Read the model definition and answer for the solid it produces. Units are mm, in the model's axes. Coordinates: 2 decimals unless noted, no trailing zeros. Order: outer loops, then holes, each group sorted by start corner. A loop starts at its lowest first (then second) coordinate and runs counter-clockwise, first axis right, second up. Notation, with made-up numbers: (-16, 62.5) -> (23, 62.5) arc R21 cw to (23, 71.5) -> close; hole circle Ø11 at (54, 34). An arc over 180 degrees is marked (long way). Return JSON: item names as keys, results as strings. Group by question number.
```python
from build123d import *

# Parameters (mm, degrees)
MODEL_R                 = 1.5
SALIENTE_EXTRUIR1_DEPTH = 3


with BuildPart() as part:
    # Model → Saliente-Extruir1 (new body)
    with BuildSketch(Plane.XY):
        with BuildLine():
            Line((-105.943383637, 101.056539338), (-105.943383637, 74.056539338))
            ThreePointArc((-105.943383637, 74.056539338), (-104.625364152, 70.874558823), (-101.443383637, 69.556539338))
            Line((-101.443383637, 69.556539338), (-20.443383637, 69.556539338))
            ThreePointArc((-20.443383637, 69.556539338), (-17.261403122, 70.874558823), (-15.943383637, 74.056539338))
            Line((-15.943383637, 74.056539338), (-15.943383637, 101.056539338))
            ThreePointArc((-15.943383637, 101.056539338), (-17.261403122, 104.238519853), (-20.443383637, 105.556539338))
            Line((-20.443383637, 105.556539338), (-101.443383637, 105.556539338))
            ThreePointArc((-101.443383637, 105.556539338), (-104.625364152, 104.238519853), (-105.943383637, 101.056539338))
        make_face()
        with Locations((-101.443383637, 101.056539338)):
            Circle(MODEL_R, mode=Mode.SUBTRACT)
        with Locations((-92.443383637, 101.056539338)):
            Circle(MODEL_R, mode=Mode.SUBTRACT)
        with Locations((-83.443383637, 101.056539338)):
            Circle(MODEL_R, mode=Mode.SUBTRACT)
        with Locations((-74.443383637, 101.056539338)):
            Circle(MODEL_R, mode=Mode.SUBTRACT)
        with Locations((-65.443383637, 101.056539338)):
            Circle(MODEL_R, mode=Mode.SUBTRACT)
        with Locations((-56.443383637, 101.056539338)):
            Circle(MODEL_R, mode=Mode.SUBTRACT)
        with Locations((-47.443383637, 101.056539338)):
            Circle(MODEL_R, mode=Mode.SUBTRACT)
        with Locations((-38.443383637, 101.056539338)):
            Circle(MODEL_R, mode=Mode.SUBTRACT)
        with Locations((-101.443383637, 92.056539338)):
            Circle(MODEL_R, mode=Mode.SUBTRACT)
        with Locations((-92.443383637, 92.056539338)):
            Circle(MODEL_R, mode=Mode.SUBTRACT)
        with Locations((-83.443383637, 92.056539338)):
            Circle(MODEL_R, mode=Mode.SUBTRACT)
        with Locations((-74.443383637, 92.056539338)):
            Circle(MODEL_R, mode=Mode.SUBTRACT)
        with Locations((-65.443383637, 92.056539338)):
            Circle(MODEL_R, mode=Mode.SUBTRACT)
        with Locations((-56.443383637, 92.056539338)):
            Circle(MODEL_R, mode=Mode.SUBTRACT)
        with Locations((-47.443383637, 92.056539338)):
            Circle(MODEL_R, mode=Mode.SUBTRACT)
        with Locations((-38.443383637, 92.056539338)):
            Circle(MODEL_R, mode=Mode.SUBTRACT)
        with Locations((-101.443383637, 83.056539338)):
            Circle(MODEL_R, mode=Mode.SUBTRACT)
        with Locations((-92.443383637, 83.056539338)):
            Circle(MODEL_R, mode=Mode.SUBTRACT)
        with Locations((-83.443383637, 83.056539338)):
            Circle(MODEL_R, mode=Mode.SUBTRACT)
        with Locations((-74.443383637, 83.056539338)):
            Circle(MODEL_R, mode=Mode.SUBTRACT)
        with Locations((-65.443383637, 83.056539338)):
            Circle(MODEL_R, mode=Mode.SUBTRACT)
        with Locations((-56.443383637, 83.056539338)):
            Circle(MODEL_R, mode=Mode.SUBTRACT)
        with Locations((-47.443383637, 83.056539338)):
            Circle(MODEL_R, mode=Mode.SUBTRACT)
        with Locations((-38.443383637, 83.056539338)):
            Circle(MODEL_R, mode=Mode.SUBTRACT)
        with Locations((-101.443383637, 74.056539338)):
            Circle(MODEL_R, mode=Mode.SUBTRACT)
        with Locations((-92.443383637, 74.056539338)):
            Circle(MODEL_R, mode=Mode.SUBTRACT)
        with Locations((-83.443383637, 74.056539338)):
            Circle(MODEL_R, mode=Mode.SUBTRACT)
        with Locations((-74.443383637, 74.056539338)):
            Circle(MODEL_R, mode=Mode.SUBTRACT)
        with Locations((-65.443383637, 74.056539338)):
            Circle(MODEL_R, mode=Mode.SUBTRACT)
        with Locations((-56.443383637, 74.056539338)):
            Circle(MODEL_R, mode=Mode.SUBTRACT)
        with Locations((-47.443383637, 74.056539338)):
            Circle(MODEL_R, mode=Mode.SUBTRACT)
        with Locations((-38.443383637, 74.056539338)):
            Circle(MODEL_R, mode=Mode.SUBTRACT)
        with Locations((-29.443383637, 101.056539338)):
            Circle(MODEL_R, mode=Mode.SUBTRACT)
        with Locations((-29.443383637, 92.056539338)):
            Circle(MODEL_R, mode=Mode.SUBTRACT)
        with Locations((-29.443383637, 83.056539338)):
            Circle(MODEL_R, mode=Mode.SUBTRACT)
        with Locations((-29.443383637, 74.056539338)):
            Circle(MODEL_R, mode=Mode.SUBTRACT)
        with Locations((-20.443383637, 101.056539338)):
            Circle(MODEL_R, mode=Mode.SUBTRACT)
        with Locations((-20.443383637, 92.056539338)):
            Circle(MODEL_R, mode=Mode.SUBTRACT)
        with Locations((-20.443383637, 83.056539338)):
            Circle(MODEL_R, mode=Mode.SUBTRACT)
        with Locations((-20.443383637, 74.056539338)):
            Circle(MODEL_R, mode=Mode.SUBTRACT)
    extrude(amount=SALIENTE_EXTRUIR1_DEPTH)


solid = part.part
```
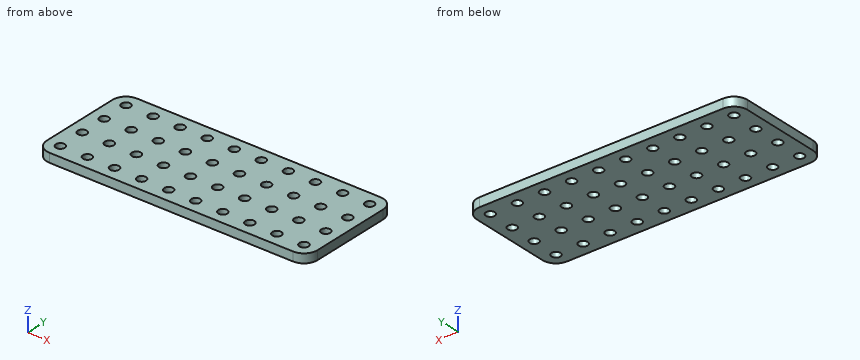
1. Find section A-A on x = -66. Determine the outline of the cut face in (y, z), and give its area (3 significant figures).
2. Find section B-B on z = 1.75. Give the number of separate pieces and of enclosed holes in the cut face, and give its area (3 significant figures).
3. Straight lines are drawn through the part: L1, parallel to Y at x = -66, z = 1.4; L2, parallel to Y at x = -46.5, z = 2.65. For each, find the intervals that lie inside material, in ascending order.
Result:
{
 "1": {"outline": "(69.56, 0) -> (72.66, 0) -> (72.66, 3) -> (69.56, 3) -> close; (75.45, 0) -> (81.66, 0) -> (81.66, 3) -> (75.45, 3) -> close; (84.45, 0) -> (90.66, 0) -> (90.66, 3) -> (84.45, 3) -> close; (93.45, 0) -> (99.66, 0) -> (99.66, 3) -> (93.45, 3) -> close; (102.45, 0) -> (105.56, 0) -> (105.56, 3) -> (102.45, 3) -> close", "area": "74.6 mm^2"},
 "2": {"separate pieces": "1", "enclosed holes": "40", "area": "2,940 mm^2"},
 "3": {"L1": "69.56 to 72.66, 75.45 to 81.66, 84.45 to 90.66, 93.45 to 99.66, 102.45 to 105.56", "L2": "69.56 to 72.89, 75.22 to 81.89, 84.22 to 90.89, 93.22 to 99.89, 102.22 to 105.56"}
}
